CAD build for the part. Positions are in the model's coordinates, mm. A direction names the side the tool comes from. Round coordinates to 2 decimals unless told otherwise and drop trailing zeros. Loops run counter-clockwise (first coordinate to the right, second up) from the corner with the lowest first, then second, coordinate; pieces in that order, holes last.
```python
from build123d import *

# Parameters (mm, degrees)
RESSALTO_EXTRUS_O2_DEPTH = 9.2
ESBO_O5_R                = 2.15
CORTE_EXTRUS_O2_DEPTH    = 9.2
CHANFRO2_SIZE            = 0.3


with BuildPart() as part:
    # Esboço4 → Ressalto-extrusão2 (new body)
    with BuildSketch(Plane(origin=(0, 0, 0), x_dir=(1, 0, 0), z_dir=(0, 1, 0))):
        with BuildLine():
            Line((-19.2, 2.35), (-19.2, 1.65))
            ThreePointArc((-19.2, 1.65), (-19.170710678, 1.579289322), (-19.1, 1.55))
            Line((-19.1, 1.55), (-18.1, 1.55))
            ThreePointArc((-18.1, 1.55), (-18.029289322, 1.579289322), (-18, 1.65))
            Line((-18, 1.65), (-18, 2.35))
            ThreePointArc((-18, 2.35), (-17.970710678, 2.420710678), (-17.9, 2.45))
            Line((-17.9, 2.45), (-17.3, 2.45))
            ThreePointArc((-17.3, 2.45), (-17.229289322, 2.420710678), (-17.2, 2.35))
            Line((-17.2, 2.35), (-17.2, 1.65))
            ThreePointArc((-17.2, 1.65), (-17.170710678, 1.579289322), (-17.1, 1.55))
            Line((-17.1, 1.55), (-16.1, 1.55))
            ThreePointArc((-16.1, 1.55), (-16.029289322, 1.579289322), (-16, 1.65))
            Line((-16, 1.65), (-16, 2.35))
            ThreePointArc((-16, 2.35), (-15.970710678, 2.420710678), (-15.9, 2.45))
            Line((-15.9, 2.45), (-15.3, 2.45))
            ThreePointArc((-15.3, 2.45), (-15.229289322, 2.420710678), (-15.2, 2.35))
            Line((-15.2, 2.35), (-15.2, 1.65))
            ThreePointArc((-15.2, 1.65), (-15.170710678, 1.579289322), (-15.1, 1.55))
            Line((-15.1, 1.55), (-14.1, 1.55))
            ThreePointArc((-14.1, 1.55), (-14.029289322, 1.579289322), (-14, 1.65))
            Line((-14, 1.65), (-14, 2.35))
            ThreePointArc((-14, 2.35), (-13.970710678, 2.420710678), (-13.9, 2.45))
            Line((-13.9, 2.45), (-13.3, 2.45))
            ThreePointArc((-13.3, 2.45), (-13.229289322, 2.420710678), (-13.2, 2.35))
            Line((-13.2, 2.35), (-13.2, 1.65))
            ThreePointArc((-13.2, 1.65), (-13.170710678, 1.579289322), (-13.1, 1.55))
            Line((-13.1, 1.55), (-12.1, 1.55))
            ThreePointArc((-12.1, 1.55), (-12.029289322, 1.579289322), (-12, 1.65))
            Line((-12, 1.65), (-12, 2.35))
            ThreePointArc((-12, 2.35), (-11.970710678, 2.420710678), (-11.9, 2.45))
            Line((-11.9, 2.45), (-11.3, 2.45))
            ThreePointArc((-11.3, 2.45), (-11.229289322, 2.420710678), (-11.2, 2.35))
            Line((-11.2, 2.35), (-11.2, 1.65))
            ThreePointArc((-11.2, 1.65), (-11.170710678, 1.579289322), (-11.1, 1.55))
            Line((-11.1, 1.55), (-10.1, 1.55))
            ThreePointArc((-10.1, 1.55), (-10.029289322, 1.579289322), (-10, 1.65))
            Line((-10, 1.65), (-10, 2.35))
            ThreePointArc((-10, 2.35), (-9.970710678, 2.420710678), (-9.9, 2.45))
            Line((-9.9, 2.45), (-9.3, 2.45))
            ThreePointArc((-9.3, 2.45), (-9.229289322, 2.420710678), (-9.2, 2.35))
            Line((-9.2, 2.35), (-9.2, 1.65))
            ThreePointArc((-9.2, 1.65), (-9.170710678, 1.579289322), (-9.1, 1.55))
            Line((-9.1, 1.55), (-8.1, 1.55))
            ThreePointArc((-8.1, 1.55), (-8.029289322, 1.579289322), (-8, 1.65))
            Line((-8, 1.65), (-8, 2.35))
            ThreePointArc((-8, 2.35), (-7.970710678, 2.420710678), (-7.9, 2.45))
            Line((-7.9, 2.45), (-7.3, 2.45))
            ThreePointArc((-7.3, 2.45), (-7.229289322, 2.420710678), (-7.2, 2.35))
            Line((-7.2, 2.35), (-7.2, 1.65))
            ThreePointArc((-7.2, 1.65), (-7.170710678, 1.579289322), (-7.1, 1.55))
            Line((-7.1, 1.55), (7.1, 1.55))
            ThreePointArc((7.1, 1.55), (7.170710678, 1.579289322), (7.2, 1.65))
            Line((7.2, 1.65), (7.2, 2.35))
            ThreePointArc((7.2, 2.35), (7.229289322, 2.420710678), (7.3, 2.45))
            Line((7.3, 2.45), (7.9, 2.45))
            ThreePointArc((7.9, 2.45), (7.970710678, 2.420710678), (8, 2.35))
            Line((8, 2.35), (8, 1.65))
            ThreePointArc((8, 1.65), (8.029289322, 1.579289322), (8.1, 1.55))
            Line((8.1, 1.55), (9.1, 1.55))
            ThreePointArc((9.1, 1.55), (9.170710678, 1.579289322), (9.2, 1.65))
            Line((9.2, 1.65), (9.2, 2.35))
            ThreePointArc((9.2, 2.35), (9.229289322, 2.420710678), (9.3, 2.45))
            Line((9.3, 2.45), (9.9, 2.45))
            ThreePointArc((9.9, 2.45), (9.970710678, 2.420710678), (10, 2.35))
            Line((10, 2.35), (10, 1.65))
            ThreePointArc((10, 1.65), (10.029289322, 1.579289322), (10.1, 1.55))
            Line((10.1, 1.55), (11.1, 1.55))
            ThreePointArc((11.1, 1.55), (11.170710678, 1.579289322), (11.2, 1.65))
            Line((11.2, 1.65), (11.2, 2.35))
            ThreePointArc((11.2, 2.35), (11.229289322, 2.420710678), (11.3, 2.45))
            Line((11.3, 2.45), (11.9, 2.45))
            ThreePointArc((11.9, 2.45), (11.970710678, 2.420710678), (12, 2.35))
            Line((12, 2.35), (12, 1.65))
            ThreePointArc((12, 1.65), (12.029289322, 1.579289322), (12.1, 1.55))
            Line((12.1, 1.55), (13.1, 1.55))
            ThreePointArc((13.1, 1.55), (13.170710678, 1.579289322), (13.2, 1.65))
            Line((13.2, 1.65), (13.2, 2.35))
            ThreePointArc((13.2, 2.35), (13.229289322, 2.420710678), (13.3, 2.45))
            Line((13.3, 2.45), (13.9, 2.45))
            ThreePointArc((13.9, 2.45), (13.970710678, 2.420710678), (14, 2.35))
            Line((14, 2.35), (14, 1.65))
            ThreePointArc((14, 1.65), (14.029289322, 1.579289322), (14.1, 1.55))
            Line((14.1, 1.55), (15.1, 1.55))
            ThreePointArc((15.1, 1.55), (15.170710678, 1.579289322), (15.2, 1.65))
            Line((15.2, 1.65), (15.2, 2.35))
            ThreePointArc((15.2, 2.35), (15.229289322, 2.420710678), (15.3, 2.45))
            Line((15.3, 2.45), (15.9, 2.45))
            ThreePointArc((15.9, 2.45), (15.970710678, 2.420710678), (16, 2.35))
            Line((16, 2.35), (16, 1.65))
            ThreePointArc((16, 1.65), (16.029289322, 1.579289322), (16.1, 1.55))
            Line((16.1, 1.55), (17.1, 1.55))
            ThreePointArc((17.1, 1.55), (17.170710678, 1.579289322), (17.2, 1.65))
            Line((17.2, 1.65), (17.2, 2.35))
            ThreePointArc((17.2, 2.35), (17.229289322, 2.420710678), (17.3, 2.45))
            Line((17.3, 2.45), (17.9, 2.45))
            ThreePointArc((17.9, 2.45), (17.970710678, 2.420710678), (18, 2.35))
            Line((18, 2.35), (18, 1.65))
            ThreePointArc((18, 1.65), (18.029289322, 1.579289322), (18.1, 1.55))
            Line((18.1, 1.55), (19.1, 1.55))
            ThreePointArc((19.1, 1.55), (19.170710678, 1.579289322), (19.2, 1.65))
            Line((19.2, 1.65), (19.2, 2.35))
            ThreePointArc((19.2, 2.35), (19.229289322, 2.420710678), (19.3, 2.45))
            Line((19.3, 2.45), (19.9, 2.45))
            ThreePointArc((19.9, 2.45), (19.970710678, 2.420710678), (20, 2.35))
            Line((20, 2.35), (20, -2.45))
            Line((20, -2.45), (-20, -2.45))
            Line((-20, -2.45), (-20, 2.35))
            ThreePointArc((-20, 2.35), (-19.970710678, 2.420710678), (-19.9, 2.45))
            Line((-19.9, 2.45), (-19.3, 2.45))
            ThreePointArc((-19.3, 2.45), (-19.229289322, 2.420710678), (-19.2, 2.35))
        make_face()
    extrude(amount=RESSALTO_EXTRUS_O2_DEPTH)

    # Esboço5 → Corte-extrusão2 (cut)
    with BuildSketch(Plane(origin=(0, 0, -1.55), x_dir=(-1, 0, 0), z_dir=(0, 0, -1))):
        with Locations((0, 4.6)):
            Circle(ESBO_O5_R)
    extrude(amount=-CORTE_EXTRUS_O2_DEPTH, mode=Mode.SUBTRACT)

    # Chanfro2
    chanfro2_edges = [part.edges().sort_by_distance(p)[0] for p in [
        (2.15, 4.6, -1.55),
    ]]
    chamfer(chanfro2_edges, length=CHANFRO2_SIZE)


solid = part.part
```
Item 1: 3-axis set-ups, long thin cutter, end or side, ignore diameter. For faces 1 (the flat face through (-18.6, 4.5, -1.55)), 2 (the flat face through (20, 5, 0)): which of +Z, -Z, +X, -X, +Y, -Y reach the whole face in a straight line?
Answers follow:
face 1: -Z, +Y, -Y
face 2: +Z, -Z, +X, +Y, -Y
Item 2: Cut at B-B, the plane z = -0.9. Give the cut face in (x, y), plus the area to 3 significant figures.
Answers follow:
outline: (-20, 0) - (20, 0) - (20, 9.2) - (-20, 9.2) - close; hole circle Ø4.3 at (0, 4.6)
area: 353 mm2
Item 3: Cut at A-A, the plane x = 0. Give the cut face in (y, z), plus the area to 3 significant figures.
Answers follow:
outline: (0, -1.55) - (2.15, -1.55) - (2.45, -1.25) - (2.45, 2.45) - (0, 2.45) - close; (6.75, -1.25) - (7.05, -1.55) - (9.2, -1.55) - (9.2, 2.45) - (6.75, 2.45) - close
area: 19.5 mm2
Item 4: Flat gauge pin, fed straight in: P1, Ø0.5, axis at x = 16.5, y = 4.5, coming from the -Z side. Where does the tip first touch, or does it go through?
Answers follow:
P1: stops at z = -1.55
Item 5: Probe line 1 (Y direction, x = 0, z = 0.25); line 2 (Z direction, x = 6, y = 5.75); line 3 (X direction, y = 5.5, z = 1.7). List the from-to ranges inside material, lowest first.
Answers follow:
line 1: y = 0 to 2.45, 6.75 to 9.2
line 2: z = -1.55 to 2.45
line 3: x = -20 to -1.95, 1.95 to 20
